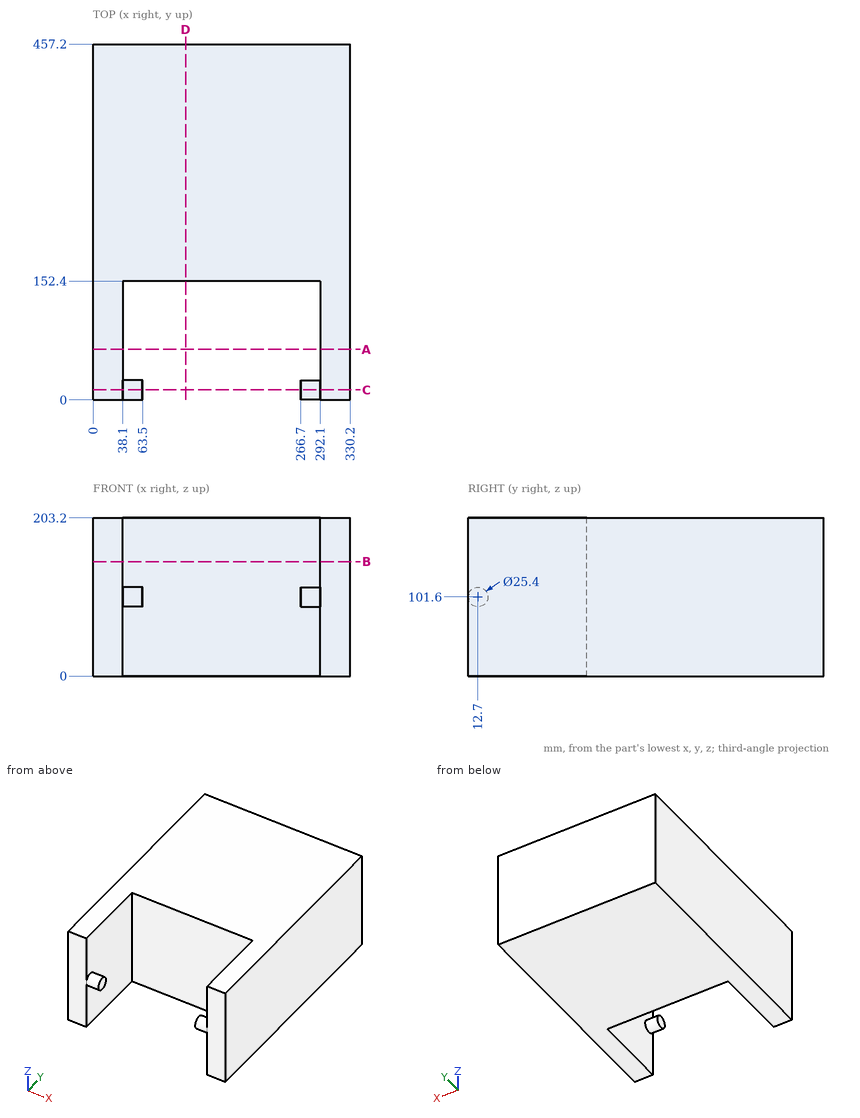
Here's the drawing with two shaded views (mm, measured from the low corner). I have some questions. Coordinates: 2 decimals unless noted, no trailing zeros. Write each loop counter-clockwise with the first axis right and the second up, starting at its lowest first coordinate (ties: lowest second). Pieces come first, ordered by that corner, then holes. Notation, with made-up numbers: M 44,10.5 L 99,10.5 A21 ccw 99,18.5 Z; hole C 89.25,68.25 d9. An arc over 180 degrees is marked long. Use one line per item in the form item = value.
Q1. If we section it at D-D (x = 119): Write out the boundary of the cut face in (y, z), then the cut area to 3 significant figures.
Model answer:
outline = M 152.4,0 L 457.2,0 L 457.2,203.2 L 152.4,203.2 Z
area = 61,900 mm^2
Q2. I need wall thicknesses on line 1 along X through (y, z) = (143, 167.5); line 2 along Y through (x, z) = (115, 63); line 3 along Y through (x, z) = (285.5, 97.5). Which ranges of each line are inside material? Lowest first, please. Write a range as from..to.
Model answer:
line_1 = 0..38.1, 292.1..330.2
line_2 = 152.4..457.2
line_3 = 0.68..24.72, 152.4..457.2
Q3. If we section it at B-B (z = 147): Write out the boundary of the cut face in (x, y), then the cut area to 3 significant figures.
Model answer:
outline = M 0,0 L 38.1,0 L 38.1,152.4 L 292.1,152.4 L 292.1,0 L 330.2,0 L 330.2,457.2 L 0,457.2 Z
area = 112,000 mm^2
Q4. If we section it at A-A (y = 65): Write out the boundary of the cut face in (x, z).
Model answer:
outline = M 0,0 L 38.1,0 L 38.1,203.2 L 0,203.2 Z; M 292.1,0 L 330.2,0 L 330.2,203.2 L 292.1,203.2 Z
Q5. If we section it at C-C (y = 12.7): Write out the boundary of the cut face in (x, z), then the cut area to 3 significant figures.
Model answer:
outline = M 0,0 L 38.1,0 L 38.1,88.9 L 63.5,88.9 L 63.5,114.3 L 38.1,114.3 L 38.1,203.2 L 0,203.2 Z; M 266.7,88.9 L 292.1,88.9 L 292.1,0 L 330.2,0 L 330.2,203.2 L 292.1,203.2 L 292.1,114.3 L 266.7,114.3 Z
area = 16,800 mm^2
